from build123d import *

# Parameters (mm, degrees)
SKETCH5_W           = 6.35
SKETCH5_H           = 118.538155393
BOSS_EXTRUDE1_DEPTH = 95.25
SKETCH7_W           = 6.35
SKETCH7_H           = 12.7
CUT_EXTRUDE1_DEPTH  = 7.35
LPATTERN1_COUNT     = 5
LPATTERN1_PITCH     = 25.4
SKETCH8_W           = 6.35
SKETCH8_H           = 12.7
CUT_EXTRUDE2_DEPTH  = 7.35
LPATTERN2_COUNT     = 5
LPATTERN2_PITCH     = 25.4
CUT_EXTRUDE3_DEPTH  = 15.875
SKETCH10_W          = 12.7
SKETCH10_H          = 6.35
SKETCH10_W_2        = 15.875
CUT_EXTRUDE4_DEPTH  = 7.35
SKETCH11_W          = 6.35
SKETCH11_H          = 6.3881
SKETCH11_W_2        = 15.875
CUT_EXTRUDE5_DEPTH  = 7.35
SKETCH13_W          = 6.35
SKETCH13_H          = 2.311210988
SKETCH13_H_2        = 2.900340521
CUT_EXTRUDE6_DEPTH  = 15.875


with BuildPart() as part:
    # Sketch5 → Boss-Extrude1 (new body)
    with BuildSketch(Plane.XY):
        with Locations((60.833541785, 251.880922304)):
            Rectangle(SKETCH5_W, SKETCH5_H)
    extrude(amount=BOSS_EXTRUDE1_DEPTH)

    # Sketch7 → Cut-Extrude1 (cut, through all)
    with BuildSketch(Plane(origin=(64.008541785, 0, 0), x_dir=(0, 0, -1), z_dir=(1, 0, 0))):
        with Locations((-92.075, 298.45)):
            Rectangle(SKETCH7_W, SKETCH7_H)
        with Locations((-3.175, 298.45)):
            Rectangle(SKETCH7_W, SKETCH7_H)
    cut_extrude1 = extrude(amount=-CUT_EXTRUDE1_DEPTH, mode=Mode.SUBTRACT)

    # LPattern1: Cut-Extrude1 ×5
    with Locations(*[(0, -i * LPATTERN1_PITCH, 0) for i in range(1, LPATTERN1_COUNT)]):
        add(cut_extrude1, mode=Mode.SUBTRACT)

    # Sketch8 → Cut-Extrude2 (cut, through all)
    with BuildSketch(Plane(origin=(64.008541785, 0, 0), x_dir=(0, 0, -1), z_dir=(1, 0, 0))):
        with Locations((-34.925, 311.15)):
            Rectangle(SKETCH8_W, SKETCH8_H)
    cut_extrude2 = extrude(amount=-CUT_EXTRUDE2_DEPTH, mode=Mode.SUBTRACT)

    # LPattern2: Cut-Extrude2 ×5
    with Locations(*[(0, -i * LPATTERN2_PITCH, 0) for i in range(1, LPATTERN2_COUNT)]):
        add(cut_extrude2, mode=Mode.SUBTRACT)

    # Sketch9 → Cut-Extrude3 (cut)
    with BuildSketch(Plane(origin=(0, 0, 0), x_dir=(-1, 0, 0), z_dir=(0, 0, -1))):
        with BuildLine():
            Line((-42.140789022, 277.931008412), (-81.069773467, 292.1))
            Line((-81.069773467, 292.1), (-81.069773467, 237.646932857))
            Line((-81.069773467, 237.646932857), (-41.263032712, 255.828523916))
            ThreePointArc((-41.263032712, 255.828523916), (-34.286165861, 267.174267761), (-42.140789022, 277.931008412))
        make_face()
    extrude(amount=-CUT_EXTRUDE3_DEPTH, mode=Mode.SUBTRACT)

    # Sketch10 → Cut-Extrude4 (cut, through all)
    with BuildSketch(Plane(origin=(64.008541785, 0, 0), x_dir=(0, 0, -1), z_dir=(1, 0, 0))):
        with Locations((-88.9, 307.975)):
            Rectangle(SKETCH10_W, SKETCH10_H)
        with Locations((-61.9125, 307.975)):
            Rectangle(SKETCH10_W_2, SKETCH10_H)
        with Locations((-33.3375, 307.975)):
            Rectangle(SKETCH10_W_2, SKETCH10_H)
        with Locations((-6.35, 307.975)):
            Rectangle(SKETCH10_W, SKETCH10_H)
    extrude(amount=-CUT_EXTRUDE4_DEPTH, mode=Mode.SUBTRACT)

    # Sketch11 → Cut-Extrude5 (cut, through all)
    with BuildSketch(Plane(origin=(64.008541785, 0, 0), x_dir=(0, 0, -1), z_dir=(1, 0, 0))):
        with Locations((-85.725, 195.805894607)):
            Rectangle(SKETCH11_W, SKETCH11_H)
        with Locations((-61.9125, 195.805894607)):
            Rectangle(SKETCH11_W_2, SKETCH11_H)
        with Locations((-33.3375, 195.805894607)):
            Rectangle(SKETCH11_W_2, SKETCH11_H)
        with Locations((-9.525, 195.805894607)):
            Rectangle(SKETCH11_W, SKETCH11_H)
    extrude(amount=-CUT_EXTRUDE5_DEPTH, mode=Mode.SUBTRACT)

    # Sketch13 → Cut-Extrude6 (cut)
    with BuildSketch(Plane(origin=(0, 0, 0), x_dir=(-1, 0, 0), z_dir=(0, 0, -1))):
        with Locations((-60.833541785, 284.734614014)):
            Rectangle(SKETCH13_W, SKETCH13_H)
        with Locations((-60.833541785, 246.889761636)):
            Rectangle(SKETCH13_W, SKETCH13_H_2)
    extrude(amount=-CUT_EXTRUDE6_DEPTH, mode=Mode.SUBTRACT)


solid = part.part
Input: part model. Units: mm. Frame: model coordinates. A direction names the side the tool comes from. Give positions to 0.01 mm unless a question says otherwise; leave off trailing zeros. Loops run counter-clockwise (first coordinate to the right, second up) from the corner with the lowest first, then second, coordinate; pieces in that order, holes last. Notation, with made-up numbers: M -25,11.5 L -15,11.5 A18 cw -15,41.5 Z; hole C 7,72.5 d4. An arc over 180 degrees is marked long. Use one line per item in the form item = value.
1. Section query B-B, the plane z = 11. Return the cut outline in (x, y).
Numbers:
outline = M 57.66,199 L 64.01,199 L 64.01,245.44 L 57.66,245.44 Z; M 57.66,285.89 L 64.01,285.89 L 64.01,304.8 L 57.66,304.8 Z
2. First-contact query: pin 1 (3 mm diameter, centred on x = 60.5, y = 195, fed in from +Z); pin 2 (1.9 mm diameter, centred on x = 61.5, y = 308, fed in from -Z); pin 3 (3 mm diameter, centred on x = 59.5, z = 3, fed in from +Y). Flat tips, straight axial feed; report the tip coordinate or a pass-through.
Numbers:
pin_1 = 82.55
pin_2 = 12.7
pin_3 = 292.1
3. Reachability of faces 1 (the face through (61, 199, 86)), 2 (the face through (61, 260, 31.75)), 3 (the face through (61, 292.1, 3)), 4 (the face through (61, 243, 6.35)), 5 (the face through (61, 241.3, 92)) from +Z, -Z, +X, -X, +Y, -Y: full face, straight path, thin tool, end or side. Return the list, or none.
Numbers:
face_1 = +Z, +X, -X, -Y
face_2 = +X, -X
face_3 = -Z, +X, -X, +Y
face_4 = -Z, +X, -X
face_5 = +Z, +X, -X
4. Line query: L1, parallel to Z at x = 61, y = 205; L2, parallel to Z at x = 62.5, y = 285 (3 decimals); L3, parallel to Y at x = 61.5, z = 13. Output: solid intervals per line, ascending.
Numbers:
L1 = 0 to 31.75, 38.1 to 95.25
L2 = 15.875 to 31.75, 38.1 to 95.25
L3 = 192.61 to 245.44, 285.89 to 311.15
5. Section query A-A, the plane y = 264. Return the cut outline in (x, z) (3 decimals).
Numbers:
outline = M 57.659,15.875 L 64.009,15.875 L 64.009,31.75 L 57.659,31.75 Z; M 57.659,38.1 L 64.009,38.1 L 64.009,95.25 L 57.659,95.25 Z
6. Section query C-C, the plane x = 61. Count the separate pieces of the cut face and the enclosed holes in it, and give its area (3 significant figures).
Numbers:
separate_pieces = 1
enclosed_holes = 4
area = 9,030 mm²
7. Section query D-D, the plane z = 64. Return the cut outline in (x, y).
Numbers:
outline = M 57.66,199 L 64.01,199 L 64.01,304.8 L 57.66,304.8 Z
8. Pull-direction query (Z, two-part tool) for faces 6 (the face through (61, 196, 82.55)), 7 (the face through (61, 279.4, 35)), 8 (the face through (61, 228.6, 35)), 9 (the face through (61, 199, 10)); classes: released by +Z, released by -Z, zero draft, split by the parting line, or undercut.
Numbers:
face_6 = released by +Z
face_7 = undercut
face_8 = undercut
face_9 = zero draft
